CAD build for the part. Positions are in the model's coordinates, mm. A direction names the side the tool comes from. Round coordinates to 2 decimals unless told otherwise and drop trailing zeros. Order: outer loops, then holes, each group sorted by start corner. A loop starts at its lowest first (then second) coordinate and runs counter-clockwise, first axis right, second up. Notation, with made-up numbers: M -17,18 L 28,18 A24 cw 28,41 Z; hole C -13.75,78.5 d9. An arc over 180 degrees is marked long. Answer as a JSON object with one key per item and string values.
```python
from build123d import *

# Parameters (mm, degrees)
SKETCH1_R           = 5
BOSS_EXTRUDE1_DEPTH = 34.5
CUT_EXTRUDE1_START  = -10
SKETCH2_R           = 5
SKETCH2_R_2         = 3
CUT_EXTRUDE1_DEPTH  = 2
CUT_EXTRUDE4_START  = -3.5
CUT_EXTRUDE4_DEPTH  = 3.2
CHAMFER1_SIZE       = 0.5
SKETCH4_OUTSIDE_W   = 26.086
SKETCH4_OUTSIDE_H   = 26.086
SKETCH4_OUTSIDE_R   = 4
CUT_EXTRUDE5_DEPTH  = 8
CHAMFER2_SIZE       = 0.5
CUT_EXTRUDE6_START  = -8
SKETCH6_OUTSIDE_W   = 26.086
SKETCH6_OUTSIDE_H   = 26.086
SKETCH6_OUTSIDE_R   = 3
CUT_EXTRUDE6_DEPTH  = 2


with BuildPart() as part:
    # Sketch1 → Boss-Extrude1 (new body, symmetric)
    with BuildSketch(Plane(origin=(0, 0, 0), x_dir=(0, 0, -1), z_dir=(1, 0, 0))):
        Circle(SKETCH1_R)
    extrude(amount=BOSS_EXTRUDE1_DEPTH, both=True)

    # Sketch2 → Cut-Extrude1 (cut)
    with BuildSketch(Plane(origin=(34.5, 0, 0), x_dir=(0, 0, -1), z_dir=(1, 0, 0)).offset(CUT_EXTRUDE1_START)):
        Circle(SKETCH2_R)
        Circle(SKETCH2_R_2, mode=Mode.SUBTRACT)
    extrude(amount=-CUT_EXTRUDE1_DEPTH, mode=Mode.SUBTRACT)

    # Sketch3 → Cut-Extrude4 (cut)
    with BuildSketch(Plane.XY.offset(CUT_EXTRUDE4_START)):
        with BuildLine():
            Line((68.42289795, -1.5), (9, -1.5))
            ThreePointArc((9, -1.5), (7.5, 0), (9, 1.5))
            Line((9, 1.5), (68.42289795, 1.5))
            Line((68.42289795, 1.5), (68.42289795, -1.5))
        make_face()
    extrude(amount=-CUT_EXTRUDE4_DEPTH, mode=Mode.SUBTRACT)

    # Chamfer1
    chamfer1_edges = [part.edges().sort_by_distance(p)[0] for p in [
        (-34.5, 0, 5),
    ]]
    chamfer(chamfer1_edges, length=CHAMFER1_SIZE)

    # Sketch4 outside → Cut-Extrude5 (cut)
    with BuildSketch(Plane.ZY.offset(34.5)):
        Rectangle(SKETCH4_OUTSIDE_W, SKETCH4_OUTSIDE_H)
        Circle(SKETCH4_OUTSIDE_R, mode=Mode.SUBTRACT)
    extrude(amount=-CUT_EXTRUDE5_DEPTH, mode=Mode.SUBTRACT)

    # Chamfer2
    chamfer2_edges = [part.edges().sort_by_distance(p)[0] for p in [
        (-34.5, 0, -4),
    ]]
    chamfer(chamfer2_edges, length=CHAMFER2_SIZE)

    # Sketch6 outside → Cut-Extrude6 (cut)
    with BuildSketch(Plane.ZY.offset(34.5).offset(CUT_EXTRUDE6_START)):
        Rectangle(SKETCH6_OUTSIDE_W, SKETCH6_OUTSIDE_H)
        Circle(SKETCH6_OUTSIDE_R, mode=Mode.SUBTRACT)
    extrude(amount=-CUT_EXTRUDE6_DEPTH, mode=Mode.SUBTRACT)


solid = part.part
```
Item 1: Saw through at C-C on x = -4.5. List the corners of the cut face in (y, z), and give its area (3 significant figures).
Worked answers:
{"outline": "C 0,0 d10", "area": "78.5 mm2"}
Item 2: Two-plate mould, pull along X, no slides. Class faces 6 (the cylindrical face through (-26, 0, -3)), 7 (the flat face through (15, 0, -3.5)), 8 (the flat face through (-34.5, 0, 0)), 9 (the flat face through (-26.5, 3, 1)): released by +X, released by -X, zero draft, split by the parting line, or undercut.
Worked answers:
{"face 6": "undercut", "face 7": "zero draft", "face 8": "released by -X", "face 9": "undercut"}
Item 3: 3-axis set-ups, long thin cutter, end or side, ignore diameter. For faces 1 (the cylindrical face through (-0.67, -4.88, 1.08)), 2 (the flat face through (24.5, -2.2, 2.4)), 3 (the flat face through (34.5, 0, 0)), 4 (the cylindrical face through (-30.303, -3.905, -0.867)), 5 (the flat face through (16, 1.5, -4)): which of +Z, -Z, +X, -X, +Y, -Y reach the whole face in a straight line?
Worked answers:
{"face 1": "+X, -X", "face 2": "none", "face 3": "+Z, -Z, +X, +Y, -Y", "face 4": "-X", "face 5": "-Z, +X"}
Item 4: Drop flat-ended pins along their axis: pin 1 Ø5 at (x, y) = (22.5, -1) entering from -Z; pin 2 Ø1.5 at (x, y) = (13.5, 0.5) entering from -Z; pin 3 Ø3 at (x, y) = (-23.5, 3) entering from +Z. Give the stop position or say it passes through.
Worked answers:
{"pin 1": "stops at z = -4.77", "pin 2": "stops at z = -3.5", "pin 3": "stops at z = 4.77"}
Item 5: Saw through at A-A on z = 0. List the corners of the cut face in (x, y).
Worked answers:
{"outline": "M -34.5,-3.5 L -34,-4 L -26.5,-4 L -26.5,-3 L -24.5,-3 L -24.5,-5 L 22.5,-5 L 22.5,-3 L 24.5,-3 L 24.5,-5 L 34.5,-5 L 34.5,5 L 24.5,5 L 24.5,3 L 22.5,3 L 22.5,5 L -24.5,5 L -24.5,3 L -26.5,3 L -26.5,4 L -34,4 L -34.5,3.5 Z"}
Item 6: Saw through at B-B on y = 0. List the corners of the cut face in (x, z).
Worked answers:
{"outline": "M -34.5,-3.5 L -34,-4 L -26.5,-4 L -26.5,-3 L -24.5,-3 L -24.5,-5 L 7.5,-5 L 7.5,-3.5 L 22.5,-3.5 L 22.5,-3 L 24.5,-3 L 24.5,-3.5 L 34.5,-3.5 L 34.5,5 L 24.5,5 L 24.5,3 L 22.5,3 L 22.5,5 L -24.5,5 L -24.5,3 L -26.5,3 L -26.5,4 L -34,4 L -34.5,3.5 Z"}
Item 7: Wall check: line 1 along X through (y, z) = (-0.25, 4.5); line 2 along X through (y, z) = (3.5, -1.25); line 3 along Z through (x, y) = (-14, 4). Give the ranges that are in metal, low to high. Write a range as [from, to].
Worked answers:
{"line 1": "x = [-24.5, 22.5], [24.5, 34.5]", "line 2": "x = [-34.28, -26.5], [-24.5, 22.5], [24.5, 34.5]", "line 3": "z = [-3, 3]"}
